The listing builds one solid part. Answer for the finished solid, in the listing's coordinates (mm). Give positions to 0.01 mm unless a question says otherwise; leave off trailing zeros. Write each loop counter-clockwise with the first axis right and the second up, starting at its lowest first coordinate (ties: lowest second). Pieces come first, ordered by that corner, then holes. Notation, with made-up numbers: (87.5, -15.5) - (91.5, -15.5) arc R21 ccw to (91.5, 2.5) - close; hole circle Ø10 at (60.25, 72). An arc over 180 degrees is marked (long way). One line per item, written item: value. Start each with the question number.
from build123d import *

# Parameters (mm, degrees)
EXTRUDE_1_DEPTH = 1


with BuildPart() as part:
    # 草图1 → 凸台-拉伸1 (new body)
    with BuildSketch(Plane(origin=(-61.5, 0, 0), x_dir=(0, -1, 0), z_dir=(-1, 0, 0))):
        with BuildLine():
            Line((145.112990447, 800.603209432), (176.378367534, 797.698696456))
            ThreePointArc((176.378367534, 797.698696456), (177.840703349, 798.15115608), (178.554793652, 799.505120921))
            Line((178.554793652, 799.505120921), (187.157332086, 892.106397006))
            Line((187.157332086, 892.106397006), (-47.830852387, 913.936494537))
            Line((-47.830852387, 913.936494537), (-56.433390821, 821.335218452))
            ThreePointArc((-56.433390821, 821.335218452), (-55.980931196, 819.872882636), (-54.626966355, 819.158792334))
            Line((-54.626966355, 819.158792334), (-23.361589268, 816.254279357))
            ThreePointArc((-23.361589268, 816.254279357), (-17.376417442, 821.221946637), (-12.408750162, 815.236774811))
            Line((-12.408750162, 815.236774811), (20.848052217, 812.147261008))
            Line((20.848052217, 812.147261008), (25.288072054, 859.941468019))
            Line((25.288072054, 859.941468019), (26.482927229, 859.830467523))
            Line((26.482927229, 859.830467523), (22.042907393, 812.036260512))
            Line((22.042907393, 812.036260512), (55.399281036, 808.937496668))
            ThreePointArc((55.399281036, 808.937496668), (61.384452862, 813.905163948), (66.352120143, 807.919992122))
            Line((66.352120143, 807.919992122), (99.708493786, 804.821228277))
            Line((99.708493786, 804.821228277), (104.148513623, 852.615435289))
            Line((104.148513623, 852.615435289), (105.343368798, 852.504434793))
            Line((105.343368798, 852.504434793), (100.903348961, 804.710227781))
            Line((100.903348961, 804.710227781), (134.16015134, 801.620713978))
            ThreePointArc((134.16015134, 801.620713978), (140.145323166, 806.588381259), (145.112990447, 800.603209432))
        make_face()
    extrude(amount=-EXTRUDE_1_DEPTH)


solid = part.part
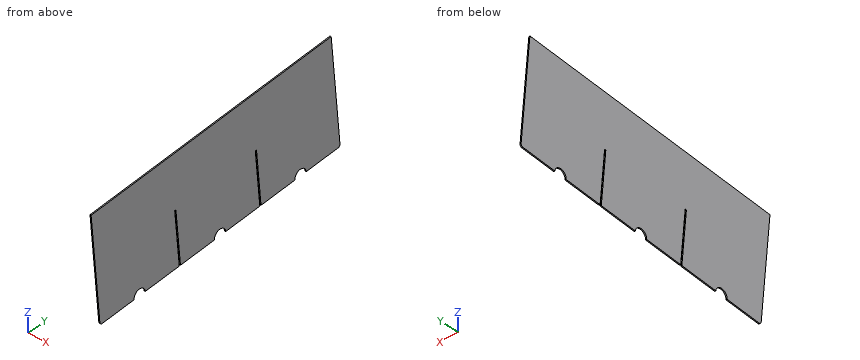
Item 1: Find section D-D on z = 870. Determine the outline of the cut face in (x, y), plus the area to 3 significant figures.
Item 2: Find section C-C on y = -160. Determine the outline of the cut face in (x, z).
Item 3: Straight lines are drawn through the part: line 1 along Y through (x, z) = (-61, 846); line 2 along Y through (x, z) = (-61.2, 829.5); line 3 along Y through (x, z) = (-60.6, 857). For each, find the intervals that lie inside material, in ascending order.
Item 4: Find section A-A on z = 829. Determine the outline of the cut face in (x, y).
Item 5: Find section B-B on x = -61. Determine the outline of the cut face in (y, z).
Values:
1. outline: (-61.5, -185.1) - (-60.5, -185.1) - (-60.5, 51.91) - (-61.5, 51.91) - close
1. area: 237 mm^2
2. outline: (-61.5, 799.22) - (-60.5, 799.22) - (-60.5, 894.63) - (-61.5, 894.63) - close
3. line 1: -182.87 to -104.74, -103.53 to -25.2, -23.99 to 54.14
3. line 2: -181.34 to -103.21, -102 to -23.67, -22.46 to 55.67
3. line 3: -183.9 to -26.22, -25.01 to 53.12
4. outline: (-61.5, -181.29) - (-60.5, -181.29) - (-60.5, -103.16) - (-61.5, -103.16) - close; (-61.5, -101.95) - (-60.5, -101.95) - (-60.5, -23.62) - (-61.5, -23.62) - close; (-61.5, -22.41) - (-60.5, -22.41) - (-60.5, 55.72) - (-61.5, 55.72) - close
5. outline: (-187.16, 892.11) - (-178.55, 799.51) arc R2 ccw to (-176.38, 797.7) - (-145.11, 800.6) arc R5.5 cw to (-134.16, 801.62) - (-100.9, 804.71) - (-105.34, 852.5) - (-104.15, 852.62) - (-99.71, 804.82) - (-66.35, 807.92) arc R5.5 cw to (-55.4, 808.94) - (-22.04, 812.04) - (-26.48, 859.83) - (-25.29, 859.94) - (-20.85, 812.15) - (12.41, 815.24) arc R5.5 cw to (23.36, 816.25) - (54.63, 819.16) arc R2 ccw to (56.43, 821.34) - (47.83, 913.94) - close
